Source: three-view drawing plus pictorial views. Frame: mm from the lowest corner of the part. A direction names the side the tool comes from. Give positions to 0.01 mm unless a question says otherwise; leave off trailing zeros. Write each loop counter-clockwise with the first axis right and the second up, starting at its lowest first coordinate (ties: lowest second). Pieces come first, ordered by that corner, then holes. Notation, with made-up numbers: (64, 62) - (91, 62) arc R24 ccw to (91, 84) - close; hole circle Ø7 at (35.5, -39.75). An arc over 180 degrees is marked (long way). One line per question, with ' | ' between items. Start each with the question number.
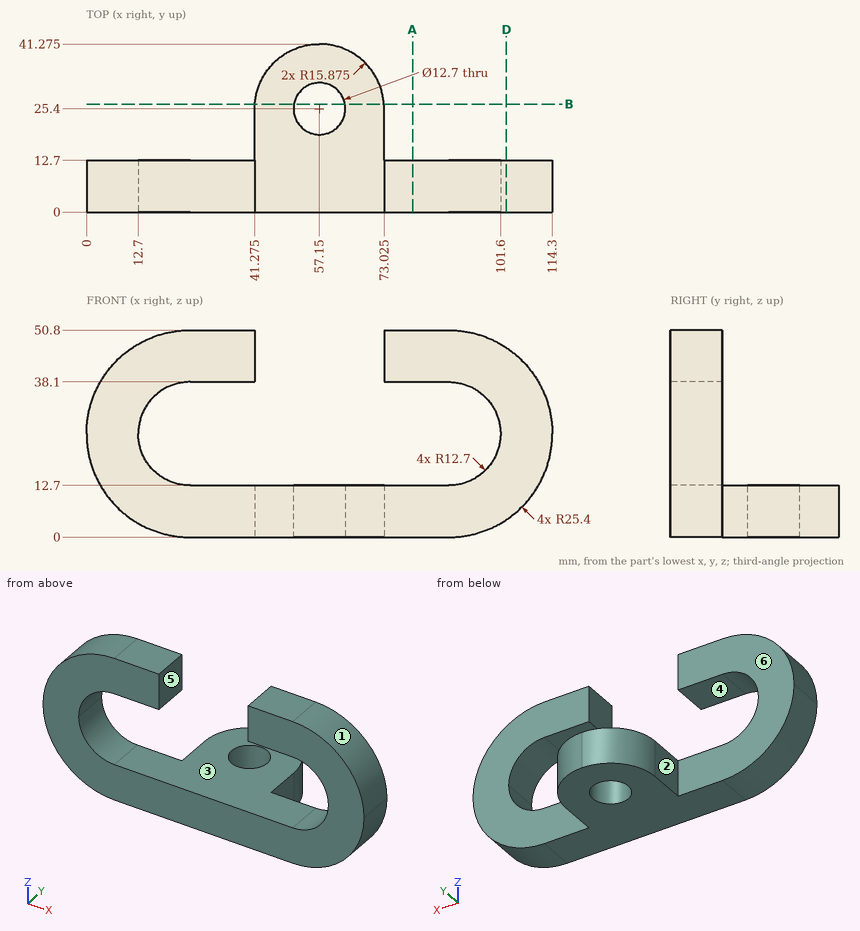
1) Line query: L1, parallel to X at y = 25, z = 7 (1 decimal); L2, parallel to Y at x = 57.15, z = 8 (3 decimals); L3, parallel to Y at x = 32, z = 45.5. Output: solid intervals per line, ascending.
2) Section A-A, the plane x = 80. Output: boundary loops of the cut face in (y, z), plus the area to 3 significant figures.
3) Pull-direction query (Z, two-part tool) for the marked faces 1, 2 and 3; classes: +Z half, -Z half, draft (parallel to the pull), parting line (faces both ways), or undercut.
4) First-contact query: pin 1 Ø4 at (y, z) = (5.5, 46) entering from -X; pin 2 Ø4 at (y, z) = (7.5, 42.5) entering from +X; pin 3 Ø6 at (y, z) = (5.5, 42) entering from -X. Flat tips, straight axial feed; report the tip coordinate or a pass-through.
5) Section D-D, the plane x = 103. Output: boundary loops of the cut face in (y, z), plus the area to 3 significant figures.
6) Section B-B, the plane y = 26.5. Output: boundary loops of the cut face in (x, z).
7) Reachability of the marked faces 4, 5 and 6 from +Z, -Z, +X, -X, +Y, -Y: full face, straight path, thin tool, end or side. Return the list, or none.
Answer key:
1) L1: 41.3 to 50.8, 63.5 to 73 | L2: 0 to 19.05, 31.75 to 41.275 | L3: 0 to 12.7
2) outline: (0, 0) - (12.7, 0) - (12.7, 12.7) - (0, 12.7) - close; (0, 38.1) - (12.7, 38.1) - (12.7, 50.8) - (0, 50.8) - close | area: 323 mm^2
3) face 1: +Z half | face 2: draft | face 3: undercut
4) pin 1: x = 8.1 | pin 2: x = 109.32 | pin 3: x = 3.95
5) outline: (0, 4.27) - (12.7, 4.27) - (12.7, 46.53) - (0, 46.53) - close | area: 537 mm^2
6) outline: (41.31, 0) - (50.9, 0) - (50.9, 12.7) - (41.31, 12.7) - close; (63.4, 0) - (72.99, 0) - (72.99, 12.7) - (63.4, 12.7) - close
7) face 4: +Y, -Y | face 5: +Z, +Y, -Y | face 6: +Z, -Z, -X, +Y
